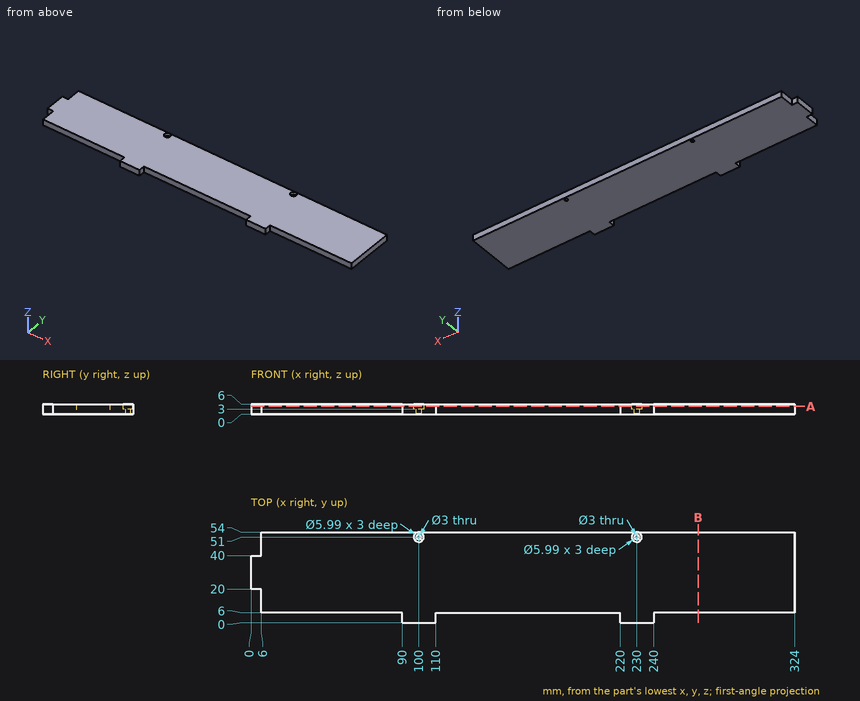
Here's the drawing with two shaded views (mm, measured from the low corner). I have some questions. Give positions to 0.01 mm unless a question says otherwise; leave off trailing zeros. Order: outer loops, then holes, each group sorted by start corner. A loop starts at its lowest first (then second) coordinate and runs counter-clockwise, first axis right, second up. Notation, with made-up numbers: (72, 76.5) -> (118, 76.5) arc R14 cw to (118, 102.5) -> close; hole circle Ø7 at (-0.75, 12.25). An arc over 180 degrees is marked (long way). Use a Markdown table: item, result. Add a question column.
Item 1: Imagine slicing it at B-B on x = 266.5. Please give me the cut outline in (y, z).
Item 2: I need wall thicknesses on line 1 (Y direction, x = 130, z = 1.45); line 2 (Y direction, x = 102, z = 5); line 3 (X direction, y = 12, z = 0.9). Which ranges of each line are inside material? Lowest first, please.
Item 3: Will these pins go through, and if not, where does the flat tip stop? pin 1 (3 mm diameter, centred on y = 3.5, z = 4, fed in from +X); pin 2 (2.5 mm diameter, centred on x = 230, y = 51, fed in from -Z); pin 3 (1.8 mm diameter, centred on y = 2, z = 2, fed in from -X); pin 4 (1.8 mm diameter, centred on y = 45.5, z = 3.5, fed in from -X).
Item 4: Imagine slicing it at A-A on z = 4.6. Please give me the cut outline in (x, y) (3 decimals).
Data:
| question | item | result |
|---|---|---|
| 1 | outline | (6, 0) -> (54, 0) -> (54, 6) -> (6, 6) -> close |
| 2 | line 1 | y = 6 to 54 |
| 2 | line 2 | y = 0 to 48.77, 53.23 to 54 |
| 2 | line 3 | x = 6 to 324 |
| 3 | pin 1 | stops at x = 240 |
| 3 | pin 2 | passes through |
| 3 | pin 3 | stops at x = 90 |
| 3 | pin 4 | stops at x = 6 |
| 4 | outline | (0, 20) -> (6, 20) -> (6, 6) -> (90, 6) -> (90, 0) -> (110, 0) -> (110, 6) -> (220, 6) -> (220, 0) -> (240, 0) -> (240, 6) -> (324, 6) -> (324, 54) -> (6, 54) -> (6, 40) -> (0, 40) -> close; hole circle Ø5.99 at (100, 51); hole circle Ø5.99 at (230, 51) |
